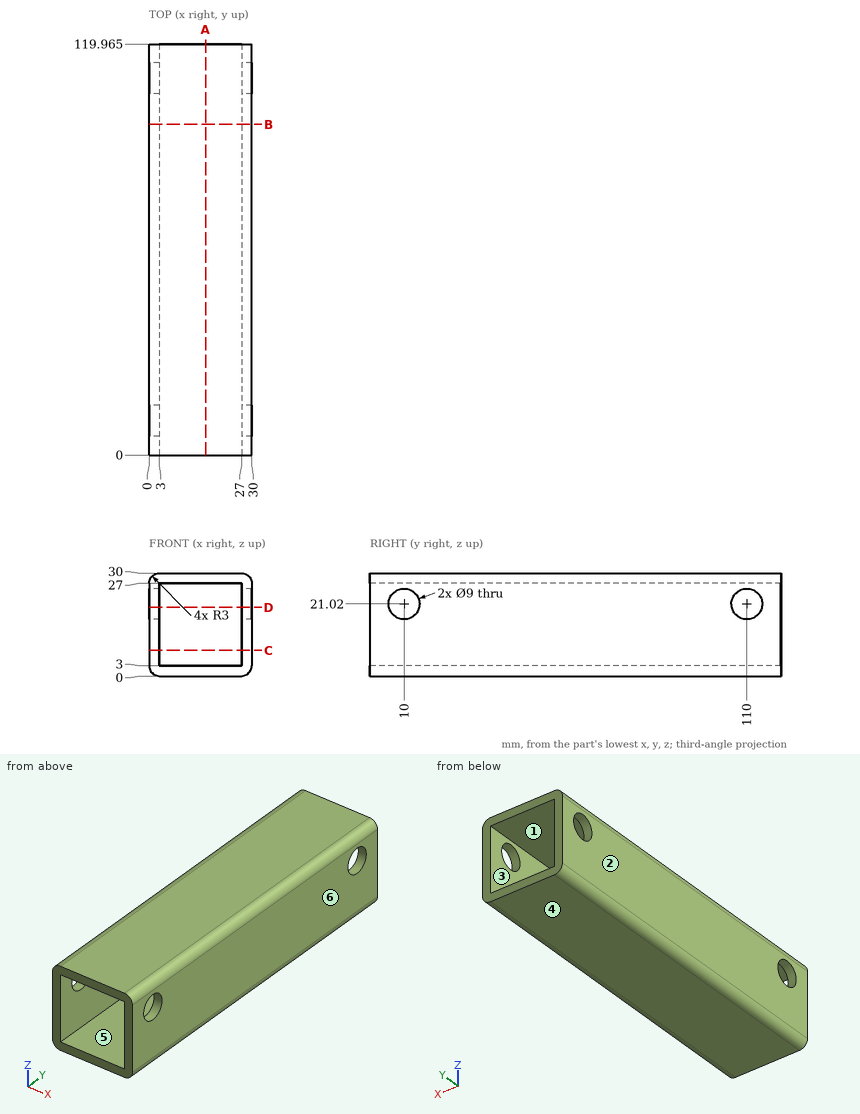
Drawing for the job (mm, zero at the part's lowest x, y, z). A direction names the side the tool comes from. Round coordinates to 2 decimals unless told otherwise and drop trailing zeros. Write each loop counter-clockwise with the first axis right and the second up, starting at its lowest first coordinate (ties: lowest second). Pieces come first, ordered by that corner, then holes. Notation, with made-up numbers: M 38.5,-19.5 L 44.5,-19.5 A18 ccw 44.5,-3.5 Z; hole C 84,-16.5 d8. An arc over 180 degrees is marked long. Answer as a JSON object with one key per item and string values. Group by question number.
(1) Cut at D-D (z = 20). Give the cut face in (x, y) (1 decimal).
(2) Drill centre lines: L1, parallel to X at y = 98, z = 8; L2, parallel to X at y = 22.5, z = 28.5. Where is each one in solid material? Low to high.
(3) Mould opens along X. For the marked faces 3, 4, 5 and 6 say: pulls with the +X half, pulls with the -X half, needs draft (parallel to the pull), parting line crosses it, or undercut.
(4) Which spindle directions (+Z, -Z, +X, -X, +Y, -Y) get a long thin tool onto all of the face, cutting with end or side? Do the marked faces 1 and 2. Say none if no direction does.
(5) Cut at A-A (x = 16.5). Give the cut face in (y, z) (1 decimal).
(6) Cut at C-C (z = 7.5). Give the cut face in (x, y) (1 decimal).
(7) Cut at B-B (y = 96.5). Give the cut face in (x, z), and give its area (3 significant figures).
(8) Flat gauge pin, fed straight in: pin 1 (1 mm diameter, centred on x = 4, z = 7, fed in from +Y). Where does the tip first touch, or does it go through?
Responses:
{
 "1": {"outline": "M 0,0 L 3,0 L 3,5.6 L 0,5.6 Z; M 0,14.4 L 3,14.4 L 3,105.6 L 0,105.6 Z; M 0,114.4 L 3,114.4 L 3,120 L 0,120 Z; M 27,0 L 30,0 L 30,5.6 L 27,5.6 Z; M 27,14.4 L 30,14.4 L 30,105.6 L 27,105.6 Z; M 27,114.4 L 30,114.4 L 30,120 L 27,120 Z"},
 "2": {"L1": "x = 0 to 3, 27 to 30", "L2": "x = 0.4 to 29.6"},
 "3": {"face 3": "undercut", "face 4": "needs draft", "face 5": "undercut", "face 6": "pulls with the +X half"},
 "4": {"face 1": "+Y, -Y", "face 2": "+Z, -Z, -X, +Y, -Y"},
 "5": {"outline": "M 0,0 L 120,0 L 120,3 L 0,3 Z; M 0,27 L 120,27 L 120,30 L 0,30 Z"},
 "6": {"outline": "M 0,0 L 3,0 L 3,120 L 0,120 Z; M 27,0 L 30,0 L 30,120 L 27,120 Z"},
 "7": {"outline": "M 0,3 A3 ccw 3,0 L 27,0 A3 ccw 30,3 L 30,27 A3 ccw 27,30 L 3,30 A3 ccw 0,27 Z; hole M 3,3 L 27,3 L 27,27 L 3,27 Z", "area": "316 mm2"},
 "8": {"pin 1": "passes through"}
}
